Input: part model. Units: mm. Frame: model coordinates. Round coordinates to 2 decimals unless told otherwise and drop trailing zeros. Order: outer loops, then holes, each group sorted by start corner. A loop starts at its lowest first (then second) coordinate and runs counter-clockwise, first axis right, second up. Notation, with made-up numbers: (35.5, 61) -> (85.5, 61) arc R26 cw to (85.5, 88) -> close; hole circle Ø11 at (4.5, 55.25). An arc over 180 degrees is marked (long way). Answer as CSV lines item,"result". Start each with the question number.
1) Section query A-A, the plane z = 0. Output: boundary loops of the cut face in (x, y).
2) Mould query, pull axis Z, two halves, no side actions, for faces 1 (the face through (-47.99, 3.13, 1.05)), 2 (the face through (7.509, 3.131, 23.846)), 3 (the face through (42, 6.35, -1)). Classes: +Z half, -Z half, draft (parallel to the pull), parting line (faces both ways), or undercut.
3) Section query C-C, the plane x = 80.5. Output: boundary loops of the cut face in (y, z), and give its area (3 significant figures).
4) Section query D-D, the plane z = -44. Output: boundary loops of the cut face in (x, y).
5) Section query B-B, the plane y = 3. State how many separate pieces and enclosed holes the cut face has, and give its area (3 significant figures).
6) Line query: L1, parallel to Z at x = -20.5, y = 4.25; L2, parallel to X at y = 0.75, z = 2; L3, parallel to X at y = 2, z = 20.35. Output: solid intervals per line, ascending.
7) First-contact query: P1, Ø2, axis at x = 85, y = 1.5, coming from the -Z side; P2, Ø1, axis at x = 47.5, y = 4.5, coming from the -Z side; P3, Ø3, axis at x = 79.5, y = 2.5, coming from the +Z side. Flat tips, straight axial feed; report the tip coordinate or a pass-through.
```python
from build123d import *

# Parameters (mm, degrees)
SKETCH1_R                 = 25
SKETCH1_R_2               = 0.5
BOSS_EXTRUDE1_DEPTH       = 6.35
M6X1_0_TAPPED_HOLE1_D     = 5
M6X1_0_TAPPED_HOLE1_DEPTH = 15
M6X1_0_TAPPED_HOLE1_TIP   = 1.502151548
M4X0_7_TAPPED_HOLE1_D     = 3.3
M4X0_7_TAPPED_HOLE1_DEPTH = 10.1
M4X0_7_TAPPED_HOLE1_TIP   = 0.991420021
FILLET1_R                 = 2


with BuildPart() as part:
    # Sketch1 → Boss-Extrude1 (new body)
    with BuildSketch(Plane(origin=(0, 0, 0), x_dir=(1, 0, 0), z_dir=(0, 1, 0))):
        with BuildLine():
            Line((100, 49.556343888), (100, -49.556343888))
            Line((100, -49.556343888), (-0.744186047, -47.994230769))
            ThreePointArc((-0.744186047, -47.994230769), (-48, 0), (-0.744186047, 47.994230769))
            Line((-0.744186047, 47.994230769), (100, 49.556343888))
        make_face()
        with Locations(Location((0, 0, 0), (0, 0, 270))):
            Circle(SKETCH1_R, mode=Mode.SUBTRACT)
        with Locations(Location((80.5, 20.35, 0), (0, 0, 270))):
            Circle(SKETCH1_R_2, mode=Mode.SUBTRACT)
        with Locations(Location((80.5, -20.35, 0), (0, 0, 270))):
            Circle(SKETCH1_R_2, mode=Mode.SUBTRACT)
        with Locations(Location((80.5, 0, 0), (0, 0, 270))):
            Circle(SKETCH1_R_2, mode=Mode.SUBTRACT)
    extrude(amount=BOSS_EXTRUDE1_DEPTH)

    # M6x1.0 Tapped Hole1
    with Locations(Plane(origin=(80.5, 6.35, -20.35), x_dir=(0, 0, 1), z_dir=(0, 1, 0))):
        with Locations((0, 0), (20.35, 0), (40.7, 0)):
            Hole(M6X1_0_TAPPED_HOLE1_D / 2, depth=M6X1_0_TAPPED_HOLE1_DEPTH)
            with Locations((0, 0, -(M6X1_0_TAPPED_HOLE1_DEPTH + M6X1_0_TAPPED_HOLE1_TIP / 2))):  # 118° drill point
                Cone(0, M6X1_0_TAPPED_HOLE1_D / 2, M6X1_0_TAPPED_HOLE1_TIP, mode=Mode.SUBTRACT)

    # M4x0.7 Tapped Hole1
    with Locations(Plane(origin=(0, 6.35, 0), x_dir=(1, 0, 0), z_dir=(0, 1, 0))):
        with Locations((-34.400585229, 27.433551282), (0, 44), (34.400585229, 27.433551282), (42.896828136, -9.790921094), (19.090884521, -39.642630188), (-19.090884521, -39.642630188), (-42.896828136, -9.790921094)):
            Hole(M4X0_7_TAPPED_HOLE1_D / 2, depth=M4X0_7_TAPPED_HOLE1_DEPTH)
            with Locations((0, 0, -(M4X0_7_TAPPED_HOLE1_DEPTH + M4X0_7_TAPPED_HOLE1_TIP / 2))):  # 118° drill point
                Cone(0, M4X0_7_TAPPED_HOLE1_D / 2, M4X0_7_TAPPED_HOLE1_TIP, mode=Mode.SUBTRACT)

    # Fillet1
    fillet1_edges = [part.edges().sort_by_distance(p)[0] for p in [
        (100, 0, 0),
        (100, 6.35, 0),
    ]]
    fillet(fillet1_edges, radius=FILLET1_R)


solid = part.part
```
Findings:
1,outline,"(-48, 0) -> (-25, 0) -> (-25, 6.35) -> (-48, 6.35) -> close; (25, 0) -> (78, 0) -> (78, 6.35) -> (25, 6.35) -> close; (83, 0) -> (98, 0) arc R2 ccw to (100, 2) -> (100, 4.35) arc R2 ccw to (98, 6.35) -> (83, 6.35) -> close"
2,face 1,"parting line"
2,face 2,"undercut"
2,face 3,"draft"
3,outline,"(0, -49.25) -> (6.35, -49.25) -> (6.35, -22.85) -> (0, -22.85) -> close; (0, -17.85) -> (6.35, -17.85) -> (6.35, -2.5) -> (0, -2.5) -> close; (0, 2.5) -> (6.35, 2.5) -> (6.35, 17.85) -> (0, 17.85) -> close; (0, 22.85) -> (6.35, 22.85) -> (6.35, 49.25) -> (0, 49.25) -> close"
3,area,"530 mm^2"
4,outline,"(-19.18, 0) -> (-1.65, 0) -> (-1.65, 6.35) -> (-19.18, 6.35) -> close; (1.65, 0) -> (98, 0) arc R2 ccw to (100, 2) -> (100, 4.35) arc R2 ccw to (98, 6.35) -> (1.65, 6.35) -> close"
5,separate pieces,"1"
5,enclosed holes,"11"
5,area,"11,300 mm^2"
6,L1,"z = -43.4 to -14.31, 14.31 to 38.78, 40.5 to 43.4"
6,L2,"x = -47.96 to -24.92, 24.92 to 79, 82 to 99.56"
6,L3,"x = -43.47 to -14.52, 14.52 to 78, 83 to 100"
7,P1,"stops at z = -49.34"
7,P2,"stops at z = -48.75"
7,P3,"stops at z = 49.26"
